Source: CAD feature listing. Evaluate the final solid. Frame: model axes, mm. A direction names the side the tool comes from. Round coordinates to 2 decimals unless told otherwise and drop trailing zeros. Loops run counter-clockwise (first coordinate to the right, second up) from the corner with the lowest first, then second, coordinate; pieces in that order, holes last.
(1) First-contact query: pin 1 Ø4 at (y, z) = (-1.5, 0.5) entering from +X; pin 2 Ø1.5 at (y, z) = (1, 4) entering from +X; pin 3 Ø1 at (x, y) = (-15, 0) entering from -Z; pin 4 Ø6 at (x, y) = (-42, -11.5) entering from -Z. Flat tips, straight axial feed; report the tip coordinate or a pass-through.
(2) Section B-B, the plane y = 0. Return the cut outline in (x, z).
(3) Section C-C, the plane x = -8. Return the cut outline in (y, z).
(4) Material intervals for probe 1 along X at (y, z) = (0, -1.5); probe 2 along Z at (x, y) = (-10.75, 0); probe 3 along Y at (x, z) = (-4, 0), sorted ascending.
(5) Set-up query: faces 1 (the flat face through (0, -0.1, 4.3)), 2 (the cylindrical face through (-1.93, 9.76, 2.17)), 3 (the cylindrical face through (-39.83, -3, -9.54)). Return all of +Z, -Z, +X, -X, +Y, -Y with unobstructed straight access to the full face (end or side cutting, diameter ignored); none if empty.
(6) Mould query, pull axis X, two halves, no side actions, for faces 4 (the flat face through (-70, 0, 0)), 5 (the cylindrical face through (-58.653, -0.766, -0.14)), 6 (the flat face through (-19, 0, 0)). Classes: pulls with the +X half, pulls with the -X half, needs draft (parallel to the pull), parting line crosses it, or undercut.
(7) Section A-A, the plane z = 0. Return the cut outline in (x, y), plus the area to 3 significant figures.
(8) Section D-D, the plane x = -60. Return the cut outline in (y, z).
```python
from build123d import *

# Parameters (mm, degrees)
CUT_EXTRUDE2_DEPTH      = 75.246212025
CUT_EXTRUDE2_DEPTH_BACK = 75.246212025
SKETCH5_R               = 2


with BuildPart() as part:
    # Sketch1 → Revolve2 (revolve)
    with BuildSketch(Plane(origin=(0, 0, 0), x_dir=(1, 0, 0), z_dir=(0, 1, 0))):
        Polygon((-3.8, 10), (-3.8, 17.5), (-8.8, 17.5), (-8.8, 10), (-70, 10), (-70, 0), (-19, 0), (-19, 4), (0, 4), (0, 10), align=None)
    revolve(axis=Axis((0, 0, 0), (-1, 0, 0)))

    # Sketch5 → Cut-Extrude2 (cut, two sides: drawn at the far end of the back side and taken through both)
    with BuildSketch(Plane.XY.offset(-CUT_EXTRUDE2_DEPTH_BACK)):
        with Locations((-39.5, 0)):
            Circle(SKETCH5_R)
        with Locations((-60.5, 0)):
            Circle(SKETCH5_R)
    extrude(amount=CUT_EXTRUDE2_DEPTH + CUT_EXTRUDE2_DEPTH_BACK, mode=Mode.SUBTRACT)


solid = part.part
```
Output values:
1. pin 1: stops at x = -19
1. pin 2: stops at x = 0
1. pin 3: stops at z = -10
1. pin 4: stops at z = -5.27
2. outline: (-70, -10) - (-62.5, -10) - (-62.5, 10) - (-70, 10) - close; (-58.5, -10) - (-41.5, -10) - (-41.5, 10) - (-58.5, 10) - close; (-37.5, -10) - (-8.8, -10) - (-8.8, -17.5) - (-3.8, -17.5) - (-3.8, -10) - (0, -10) - (0, -4) - (-19, -4) - (-19, 4) - (0, 4) - (0, 10) - (-3.8, 10) - (-3.8, 17.5) - (-8.8, 17.5) - (-8.8, 10) - (-37.5, 10) - close
3. outline: circle Ø35 at (0, 0); hole circle Ø8 at (0, 0)
4. probe 1: x = -70 to -62.5, -58.5 to -41.5, -37.5 to -19
4. probe 2: z = -10 to -4, 4 to 10
4. probe 3: y = -17.5 to -4, 4 to 17.5
5. face 1: +Z, -Z, +X, +Y, -Y
5. face 2: +X
5. face 3: -X
6. face 4: pulls with the -X half
6. face 5: undercut
6. face 6: pulls with the +X half
7. outline: (-70, -10) - (-8.8, -10) - (-8.8, -17.5) - (-3.8, -17.5) - (-3.8, -10) - (0, -10) - (0, -4) - (-19, -4) - (-19, 4) - (0, 4) - (0, 10) - (-3.8, 10) - (-3.8, 17.5) - (-8.8, 17.5) - (-8.8, 10) - (-70, 10) - close; hole circle Ø4 at (-60.5, 0); hole circle Ø4 at (-39.5, 0)
7. area: 1,300 mm2
8. outline: (-1.94, -9.81) - (-1.94, 9.81) arc R10 ccw to start; (1.94, -9.81) arc R10 ccw to (1.94, 9.81) - close
